Source: CAD feature listing. Evaluate the final solid. Frame: model axes, mm. A direction names the side the tool comes from. Give positions to 0.01 mm unless a question says otherwise; leave off trailing zeros. Write each loop counter-clockwise with the first axis right and the second up, starting at its lowest first coordinate (ties: lowest second). Pieces come first, ordered by that corner, then holes.
```python
from build123d import *

# Parameters (mm, degrees)
F0_W     = 25.4
F0_H     = 762
F1_DEPTH = 25.4
F2_W     = 25.4
F2_H     = 25.4
F3_DEPTH = 304.8
F4_W     = 25.4
F4_H     = 25.4
F5_DEPTH = 279.4


with BuildPart() as f1:
    # F0 (on Right) → F1 (new body)
    with BuildSketch(Plane.YZ):
        with Locations((7.826157, 79.498407)):
            Rectangle(F0_W, F0_H)
    extrude(amount=F1_DEPTH)

    # F2 (on face) → F3 (join)
    with BuildSketch(Plane.XZ.offset(4.873843)):
        with Locations((12.7, 447.798407)):
            Rectangle(F2_W, F2_H)
    extrude(amount=F3_DEPTH)

    # F4 (on face) → F5 (join)
    with BuildSketch(Plane(origin=(0, 0, 435.098407), x_dir=(1, 0, 0), z_dir=(0, 0, -1))):
        with Locations((12.7, 296.973843)):
            Rectangle(F4_W, F4_H)
    extrude(amount=F5_DEPTH)


solid = f1.part
```
1. Access query for faces 1 (the flat face through (13, -143, 435.098)), 2 (the flat face through (13, -297, 155.698)), 3 (the flat face through (13, -142, 460.498)). Directions: +Z, -Z, +X, -X, +Y, -Y. A direction counts if a zero-diameter tool reaches every point of the face in a straight line with its end or side. Return the directions, or none.
2. Section query A-A (z = 227). Return loops of the section in (x, y).
3. Line query: probe 1 along Y at (x, z) = (11.5, 361); probe 2 along Y at (x, z) = (5.5, -193); probe 3 along Z at (x, y) = (3.75, -48). Output: solid intervals per line, ascending.
4. Section query C-C (y = -140). Return loops of the section in (x, z), plus the area to 3 significant figures.
5. Section query D-D (z = -41). Return loops of the section in (x, y), plus the area to 3 significant figures.
6. Section query B-B (x = 5). Return loops of the section in (y, z), plus the area to 3 significant figures.
7. Pin query (flat end, axial travel): P1, Ø7.5, axis at x = 14.5, y = -294, coming from the -Z side; P2, Ø12.5, axis at x = 17.5, z = 113.5, coming from the -Y side; P3, Ø10, axis at x = 12.5, y = -59, coming from the -Z side. Return the tip coordinate at first contact, or that it passes through.
8. Pull-direction query (Y, two-part tool) for faces 4 (the flat face through (13, -4.874, 62)), 5 (the flat face through (25.4, 3, 222)), 6 (the flat face through (13, 20.526, 74)); classes: pulls with the +Y half, pulls with the -Y half, needs draft (parallel to the pull), parting line crosses it, or undercut.
The answers:
1. face 1: -Z, +X, -X
1. face 2: -Z, +X, -X, -Y
1. face 3: +Z, +X, -X, +Y, -Y
2. outline: (0, -309.67) - (25.4, -309.67) - (25.4, -284.27) - (0, -284.27) - close; (0, -4.87) - (25.4, -4.87) - (25.4, 20.53) - (0, 20.53) - close
3. probe 1: y = -309.67 to -284.27, -4.87 to 20.53
3. probe 2: y = -4.87 to 20.53
3. probe 3: z = 435.1 to 460.5
4. outline: (0, 435.1) - (25.4, 435.1) - (25.4, 460.5) - (0, 460.5) - close
4. area: 645 mm2
5. outline: (0, -4.87) - (25.4, -4.87) - (25.4, 20.53) - (0, 20.53) - close
5. area: 645 mm2
6. outline: (-309.67, 155.7) - (-284.27, 155.7) - (-284.27, 435.1) - (-4.87, 435.1) - (-4.87, -301.5) - (20.53, -301.5) - (20.53, 460.5) - (-309.67, 460.5) - close
6. area: 34,200 mm2
7. P1: stops at z = 155.7
7. P2: stops at y = -4.87
7. P3: stops at z = 435.1
8. face 4: undercut
8. face 5: needs draft
8. face 6: pulls with the +Y half
